Autodesk Inventor part; units mm, degrees
ref_plane "YZ Plane" through (0, 0, 0) normal (1, 0, 0) x (0, 1, 0)
ref_plane "XZ Plane" through (0, 0, 0) normal (0, 1, 0) x (-1, 0, 0)
ref_plane "XY Plane" through (0, 0, 0) normal (0, 0, 1) x (1, 0, 0)
sketch "Boceto1" plane through (0, 0, 0) normal (0, 1, 0) x (-1, 0, 0)
  line L0 (37.5, 25) -> (-37.5, 25)
  line L1 (-37.5, 25) -> (-37.5, -25)
  line L2 (-37.5, -25) -> (37.5, -25)
  line L3 (37.5, -25) -> (37.5, 25)
  line L4 (34, 21.5) -> (-34, 21.5) construction
  line L5 (-34, 21.5) -> (-34, -21.5) construction
  line L6 (-34, -21.5) -> (34, -21.5) construction
  line L7 (34, -21.5) -> (34, 21.5) construction
  circle A0 centre (34, 21.5) radius 1.5
  circle A1 centre (34, -21.5) radius 1.5
  circle A2 centre (-34, -21.5) radius 1.5
  circle A3 centre (-34, 21.5) radius 1.5
  point P0 (0, 0)
  point P1 (37.5, 0)
  point P2 (0, 25)
  dimension "d0" = 3
  dimension "d1" = 3.5
  dimension "d2" = 50
  dimension "d3" = 75
  dimension "d6" = 43
  dimension "d7" = 68
extrude "Extrusión1" add sketch "Boceto1" along normal blind 2
properties part number "driver motor"
Read the model definition and answer for the solid it produces. Units are mm, in the model's axes. Round coordinates to 2 decimals unless told otherwise and drop trailing zeros. Write each loop counter-clockwise with the first axis right and the second up, starting at its lowest first coordinate (ties: lowest second). Pieces come first, ordered by that corner, then holes. Notation, with made-up numbers: (-31, 9.25) - (5, 9.25) arc R13 ccw to (5, 28.25) - close; hole circle Ø11 at (16.5, 40). An arc over 180 degrees is marked (long way). One line per item, written item: value.
Q1. Find section A-A (z = 21.5). Determine the outline of the cut face in (x, y).
The answers:
outline: (-37.5, 0) - (-35.5, 0) - (-35.5, 2) - (-37.5, 2) - close; (-32.5, 0) - (32.5, 0) - (32.5, 2) - (-32.5, 2) - close; (35.5, 0) - (37.5, 0) - (37.5, 2) - (35.5, 2) - close
Q2. A straight line is drawn through the part: line 1 (Z direction, x = 34, y = 1.5). Find the intervals that lie inside material, in ascending order. Write a range as from..to.
The answers:
line 1: z = -25..-23, -20..20, 23..25
Q3. For a pull along Z with two mould halves and no side action, classify faces 1 (the flat face through (1, 0, 0)), 2 (the flat face through (1, 1, -25)), 3 (the cylindrical face through (35.11, 0.99, 20.49)) as pulls with the +Z half, pulls with the -Z half, needs draft (parallel to the pull), parting line crosses it, or undercut.
The answers:
face 1: needs draft
face 2: pulls with the -Z half
face 3: undercut
Q4. Find section B-B (x = 34). Determine the outline of the cut face in (y, z).
The answers:
outline: (0, -25) - (2, -25) - (2, -23) - (0, -23) - close; (0, -20) - (2, -20) - (2, 20) - (0, 20) - close; (0, 23) - (2, 23) - (2, 25) - (0, 25) - close
